Job drawing, mm, ordinate dimensions from the low corner. One solid piece. Round coordinates to 2 decimals unless told otherwise and drop trailing zeros. Write each loop counter-clockwise with the first axis right and the second up, starting at its lowest first coordinate (ties: lowest second). Pieces come first, ordered by that corner, then holes.
1) Saw through at C-C (y = 8.25). Write the cut outline in (x, z).
2) Saw through at B-B (z = 273). Write the cut outline in (x, y).
3) Flat gauge pins, fed straight in: pin 1 (4 mm diameter, centred on x = 257.75, z = 318.33, fed in from -Y); pin 2 (4 mm diameter, centred on x = 71, y = 4.5, fed in from -Z); pin 3 (1 mm diameter, centred on y = 5, z = 57.5, fed in from -X); pin 4 (6 mm diameter, centred on y = 6, z = 74, fed in from +X). Where does each tip first touch, or does it go through?
4) Wall check: probe 1 along Z at (x, y) = (92.25, 3.25) (1 decimal); probe 2 along Z at (x, y) = (221.5, 0.5); probe 3 along Z at (x, y) = (250, 7). Give the ranges that are in metal, low to high.
5) Saw through at A-A (x = 175). Write the cut outline in (y, z).
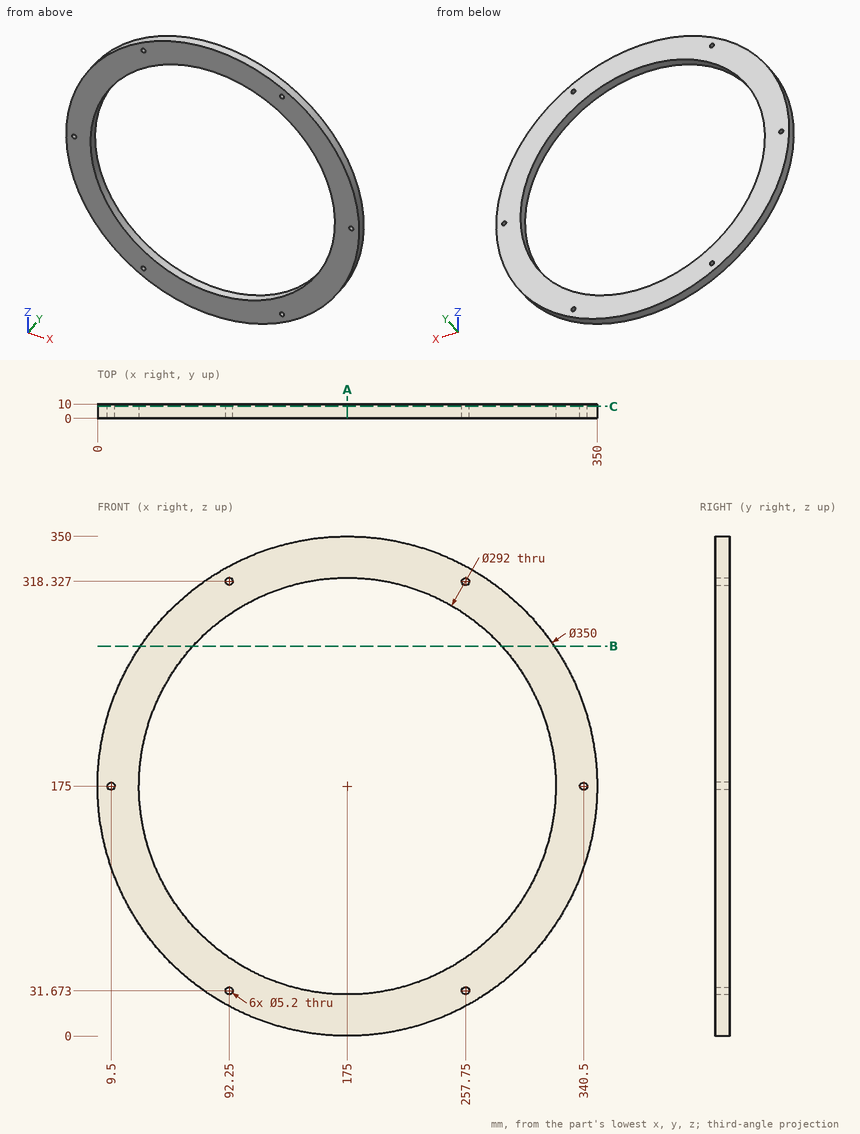
Evaluation:
1. outline: circle Ø350 at (175, 175); hole circle Ø5.2 at (9.5, 175); hole circle Ø292 at (175, 175); hole circle Ø5.2 at (92.25, 31.67); hole circle Ø5.2 at (92.25, 318.33); hole circle Ø5.2 at (257.75, 31.67); hole circle Ø5.2 at (257.75, 318.33); hole circle Ø5.2 at (340.5, 175)
2. outline: (30.01, 0) - (66.78, 0) - (66.78, 10) - (30.01, 10) - close; (283.22, 0) - (319.99, 0) - (319.99, 10) - (283.22, 10) - close
3. pin 1: passes through
3. pin 2: stops at z = 32.8
3. pin 3: stops at x = 44.86
3. pin 4: stops at x = 319.99
4. probe 1: z = 20.8 to 29.1, 34.3 to 54.7, 295.3 to 315.7, 320.9 to 329.2
4. probe 2: z = 6.29 to 36.6, 313.4 to 343.71
4. probe 3: z = 16.89 to 49.74, 300.26 to 333.11
5. outline: (0, 0) - (10, 0) - (10, 29) - (0, 29) - close; (0, 321) - (10, 321) - (10, 350) - (0, 350) - close
